Build history of the part. All positions in model axes, mm. Give positions to 0.01 mm unless a question says otherwise; leave off trailing zeros. Order: outer loops, then holes, each group sorted by start corner. A loop starts at its lowest first (then second) coordinate and runs counter-clockwise, first axis right, second up. Notation, with made-up numbers: (74.5, -15) - (89.5, -15) arc R23 cw to (89.5, 18) - close; hole circle Ø4 at (-26, 89.5). An arc over 180 degrees is marked (long way). Answer in a Markdown table with one row per item.
```python
from build123d import *

# Parameters (mm, degrees)
SKETCH_W  = 29.5
SKETCH_H  = 20.5
SKETCH_R  = 3.2
PAD_DEPTH = 7


with BuildPart() as part:
    # Sketch → Pad (new body)
    with BuildSketch(Plane.XY):
        with Locations((-14.75, 10.25)):
            Rectangle(SKETCH_W, SKETCH_H)
        with Locations((-21.5, 12.5)):
            Circle(SKETCH_R, mode=Mode.SUBTRACT)
    pad = extrude(amount=PAD_DEPTH)

    # Mirrored: Pad across Sketch V_Axis
    add(pad.mirror(Plane(origin=(0, 0, 0), x_dir=(0, 0, 1), z_dir=(1, 0, 0))))


solid = part.part
```
1. Cut at C-C on z = 6.25. Write the cut outline in (x, y).
Check result:
| item | result |
|---|---|
| outline | (-29.5, 0) - (29.5, 0) - (29.5, 20.5) - (-29.5, 20.5) - close; hole circle Ø6.4 at (-21.5, 12.5); hole circle Ø6.4 at (21.5, 12.5) |
2. Probe line 1 (Y direction, x = -21.5, z = 4.25); line 2 (X direction, y = 15, z = 5.5); line 3 (X direction, y = 10.25, z = 2.75). List the from-to ranges inside material, lowest first.
Check result:
| item | result |
|---|---|
| line 1 | y = 0 to 9.3, 15.7 to 20.5 |
| line 2 | x = -29.5 to -23.5, -19.5 to 19.5, 23.5 to 29.5 |
| line 3 | x = -29.5 to -23.78, -19.22 to 19.22, 23.78 to 29.5 |
3. Cut at A-A on y = 12.5. Write the cut outline in (x, z).
Check result:
| item | result |
|---|---|
| outline | (-29.5, 0) - (-24.7, 0) - (-24.7, 7) - (-29.5, 7) - close; (-18.3, 0) - (18.3, 0) - (18.3, 7) - (-18.3, 7) - close; (24.7, 0) - (29.5, 0) - (29.5, 7) - (24.7, 7) - close |
4. Drop a flat-ended pin along its axis: P1, Ø5, axis at x = -21.5, y = 12.5, coming from the -Z side. Give the stop position or say it passes through.
Check result:
| item | result |
|---|---|
| P1 | passes through |
5. Two-plate mould, pull along X, no slides. Class faces 1 (the face through (-24.7, 12.6, 3.5)), 2 (the face through (24.7, 12.6, 3.5)), 3 (the face through (-29.5, 10, 3)), 4 (the face through (0, 0, 3)): +X half, -X half, draft (parallel to the pull), parting line (faces both ways), or undercut.
Check result:
| item | result |
|---|---|
| face 1 | undercut |
| face 2 | undercut |
| face 3 | -X half |
| face 4 | draft |
6. Cut at B-B on x = 21.5. Write the cut outline in (y, z).
Check result:
| item | result |
|---|---|
| outline | (0, 0) - (9.3, 0) - (9.3, 7) - (0, 7) - close; (15.7, 0) - (20.5, 0) - (20.5, 7) - (15.7, 7) - close |
